Check sheet for the modelled part. Datum: model origin and axes. Units: mm. A direction names the side the tool comes from. Give positions to 0.01 mm unless a question says otherwise; leave off trailing zeros. Order: outer loops, then holes, each group sorted by start corner. A loop starts at its lowest first (then second) coordinate and runs counter-clockwise, first axis right, second up.
```python
from build123d import *

# Parameters (mm, degrees)
F0_W          = 16.5
F0_H          = 11
F1_DEPTH      = 10
F2_W          = 5
F2_H          = 11
F3_DEPTH      = 21
F4_R          = 1.1
F5_DEPTH      = 25
F6_W          = 1.5
F6_H          = 11
F7_DEPTH      = 21
F8_DEPTH      = 25.75
F9_W          = 13
F9_H          = 10
F10_DEPTH     = 10
F11_R         = 3
F12_DEPTH     = 3.5
F13_R         = 1.45
F14_DEPTH     = 25
F15_R         = 1
F16_T1_DEPTH  = 11
F16_S5_W      = 1
F16_S5_H      = 1
F16_T6_DEPTH  = 1
F16_S11_W     = 1
F16_S11_H     = 1
F16_T12_DEPTH = 1


# Not quite as in the source:
# - a fillet or chamfer that OpenCascade refuses, or shapes differently, is made with other operations: its cross-section is extruded or revolved along the edge and cut away or added


with BuildPart() as f1:
    # F0 (on Front) → F1 (new body)
    with BuildSketch(Plane.XZ):
        with Locations((8.25, 5.5)):
            Rectangle(F0_W, F0_H)
    extrude(amount=F1_DEPTH)

    # F2 (on face) → F3 (join)
    with BuildSketch(Plane.XZ.offset(10)):
        with Locations((14, 5.5)):
            Rectangle(F2_W, F2_H)
        with Locations((2.5, 5.5)):
            Rectangle(F2_W, F2_H)
    extrude(amount=F3_DEPTH)

    # F4 (on face) → F5 (cut)
    with BuildSketch(Plane(origin=(0, 0, 0), x_dir=(0, -1, 0), z_dir=(-1, 0, 0))):
        with BuildLine():
            ThreePointArc((24.9, 8), (26, 6.9), (27.1, 8))
            Line((27.1, 8), (26, 8))
            Line((26, 8), (24.9, 8))
        make_face()
        with BuildLine():
            Line((26, 8), (27.1, 8))
            ThreePointArc((27.1, 8), (26, 9.1), (24.9, 8))
            Line((24.9, 8), (26, 8))
        make_face()
        with Locations((16.5, 8)):
            Circle(F4_R)
    extrude(amount=-F5_DEPTH, mode=Mode.SUBTRACT)

    # F6 (on face) → F7 (cut)
    with BuildSketch(Plane.XZ.offset(31)):
        with Locations((0.75, 5.5)):
            Rectangle(F6_W, F6_H)
    extrude(amount=-F7_DEPTH, mode=Mode.SUBTRACT)

    # F8 (add): a face of the model
    f8_faces = [f1.faces().sort_by_distance(p)[0] for p in [
        (0, -5, 5.5),
    ]]
    extrude(f8_faces, amount=F8_DEPTH)

    # F9 (on face) → F10 (join)
    with BuildSketch(Plane.XY.offset(11)):
        with Locations((-19.25, -5)):
            Rectangle(F9_W, F9_H)
    extrude(amount=F10_DEPTH)

    # F11 (on face) → F12 (cut)
    with BuildSketch(Plane(origin=(0, 0, 0), x_dir=(-1, 0, 0), z_dir=(0, 1, 0))):
        with BuildLine():
            ThreePointArc((22.25, 15.75), (21.3713203436, 17.8713203436), (19.25, 18.75))
            Line((19.25, 18.75), (19.25, 12.75))
            ThreePointArc((19.25, 12.75), (21.3713203436, 13.6286796564), (22.25, 15.75))
        make_face()
        with BuildLine():
            Line((19.25, 12.75), (19.25, 18.75))
            ThreePointArc((19.25, 18.75), (16.25, 15.75), (19.25, 12.75))
        make_face()
        with Locations((19.25, 5.25)):
            Circle(F11_R)
    extrude(amount=-F12_DEPTH, mode=Mode.SUBTRACT)

    # F13 (on face) → F14 (cut)
    with BuildSketch(Plane(origin=(0, 0, 0), x_dir=(-1, 0, 0), z_dir=(0, 1, 0))):
        with Locations((19.25, 15.75)):
            Circle(F13_R)
        with Locations((19.25, 5.25)):
            Circle(F13_R)
    extrude(amount=-F14_DEPTH, mode=Mode.SUBTRACT)

    # F15
    f15_edges = [f1.edges().sort_by_distance(p)[0] for p in [
        (-12.75, -5, 21),
        (-25.75, -5, 21),
        (-19.25, 0, 21),
        (-25.75, 0, 10.5),
        (-25.75, -10, 10.5),
        (-25.75, -5, 0),
        (-4.625, 0, 0),
        (-12.125, -10, 0),
        (-12.75, 0, 16),
        (-12.75, -10, 16),
        (1.875, 0, 11),
        (-5.625, -10, 11),
        (8.25, -10, 11),
        (8.25, -10, 0),
        (3.25, -31, 11),
        (14, -31, 11),
        (14, -31, 0),
        (16.5, -15.5, 0),
        (3.25, -31, 0),
    ]]
    fillet(f15_edges, radius=F15_R)

    # F16: fillet of radius 1 on 1 edges, made by hand

    # F16_s2 → F16_t1 (cut)
    with BuildSketch(Plane.YZ.offset(-24.75)):
        with BuildLine():
            ThreePointArc((-10, 20), (-9.7071067812, 20.7071067812), (-9, 21))
            Line((-9, 21), (-10, 21))
            Line((-10, 21), (-10, 20))
        make_face()
    extrude(amount=F16_T1_DEPTH, mode=Mode.SUBTRACT)


with BuildPart() as f16_tool4:
    # F16_s5 → F16_t6 (new body)
    with BuildSketch(Plane.XZ.offset(9)):
        with Locations((-25.25, 20.5)):
            Rectangle(F16_S5_W, F16_S5_H)
    extrude(amount=F16_T6_DEPTH)

    # F16_s7 → F16_t8 (revolve, cut)
    with BuildSketch(Plane(origin=(-24.75, -9, 20), x_dir=(0.7071067812, 0, -0.7071067812), z_dir=(-0.7071067812, 0, -0.7071067812))):
        with BuildLine():
            ThreePointArc((0, -1), (1, 0), (0, 1))
            Line((0, 1), (0, -1))
        make_face()
    revolve(axis=Axis((-24.75, -9, 20), (0, -1, 0)), mode=Mode.SUBTRACT)


with BuildPart() as f1_1:
    add(f1.part)

    # F16_t3: cut F16_tool4
    add(f16_tool4.part, mode=Mode.SUBTRACT)


with BuildPart() as f16_tool10:
    # F16_s11 → F16_t12 (new body)
    with BuildSketch(Plane.XZ.offset(9)):
        with Locations((-13.25, 20.5)):
            Rectangle(F16_S11_W, F16_S11_H)
    extrude(amount=F16_T12_DEPTH)

    # F16_s13 → F16_t14 (revolve, cut)
    with BuildSketch(Plane(origin=(-13.75, -9, 20), x_dir=(-0.7071067812, 0, -0.7071067812), z_dir=(-0.7071067812, 0, 0.7071067812))):
        with BuildLine():
            ThreePointArc((0, -1), (1, 0), (0, 1))
            Line((0, 1), (0, -1))
        make_face()
    revolve(axis=Axis((-13.75, -9, 20), (0, -1, 0)), mode=Mode.SUBTRACT)


with BuildPart() as f1_2:
    add(f1_1.part)

    # F16_t9: cut F16_tool10
    add(f16_tool10.part, mode=Mode.SUBTRACT)


solid = f1_2.part
```
(1) Cross-section at D-D on y = -2. Enter the section's corners in (x, z), then the cut area to 3 significant figures.
Response values:
outline: (-25.75, 1) arc R1 ccw to (-24.75, 0) - (15.5, 0) arc R1 ccw to (16.5, 1) - (16.5, 11) - (-12.75, 11) - (-12.75, 20) arc R1 ccw to (-13.75, 21) - (-24.75, 21) arc R1 ccw to (-25.75, 20) - close; hole circle Ø6 at (-19.25, 5.25); hole circle Ø6 at (-19.25, 15.75)
area: 537 mm2
(2) Release check for a two-part mould opening along Y. For faces 4 (the face through (3.274, -30.699, 10.715)), 5 (the face through (3.23, -15.63, 7.33)), 6 (the face through (-21, -3.5, 6)) record: released by +Y, released by -Y, zero draft, split by the parting line, or undercut.
Response values:
face 4: released by -Y
face 5: undercut
face 6: released by +Y
(3) Cross-section at A-A on z = 5.25. Enter the section's corners in (x, y).
Response values:
outline: (-25.75, -9) arc R1 ccw to (-24.75, -10) - (-20.7, -10) - (-20.7, -3.5) - (-22.25, -3.5) - (-22.25, 0) - (-24.75, 0) arc R1 ccw to (-25.75, -1) - close; (-17.8, -10) - (1.5, -10) - (1.5, -31) - (5, -31) - (5, -10) - (11.5, -10) - (11.5, -31) - (16.5, -31) - (16.5, 0) - (-16.25, 0) - (-16.25, -3.5) - (-17.8, -3.5) - close
(4) Gauge pin test, flat ends, axial feed: pin 1 Ø1.5 at (x, z) = (-2.5, 12) entering from +Y; pin 2 Ø12 at (y, z) = (-15.5, 2.5) entering from -X; pin 3 Ø12 at (x, y) = (7, -17) entering from +Z; pin 4 Ø3 at (x, z) = (8.5, 7) entering from -Y. Record the tip position at first contact, or that the pin passes through.
Response values:
pin 1: passes through
pin 2: stops at x = -25.62
pin 3: stops at z = 11
pin 4: stops at y = -10
(5) Cross-section at C-C on x = 3.5. Enter the section's corners in (y, z), then the cut area to 3 significant figures.
Response values:
outline: (-31, 1) arc R1 ccw to (-30, 0) - (-1, 0) arc R1 ccw to (0, 1) - (0, 10) arc R1 ccw to (-1, 11) - (-30, 11) arc R1 ccw to (-31, 10) - close; hole circle Ø2.2 at (-26, 8); hole circle Ø2.2 at (-16.5, 8)
area: 333 mm2
(6) Set-up check for faces 1 (the face through (5.33, -8.85, 11)), 2 (the face through (8.296, -9.699, 0.285)), 3 (the face through (-13.051, -0.285, 15.07)): record each of +Z, -Z, +X, -X, +Y, -Y from which the full face is reachable in a straight line by a thin tool's end or side.
Response values:
face 1: +Z, +X, +Y, -Y
face 2: -Z, -Y
face 3: +Z, +X, +Y
(7) Cross-section at B-B on y = -26. Enter the section's corners in (x, z).
Response values:
outline: (1.5, 0) - (5, 0) - (5, 6.9) - (1.5, 6.9) - close; (1.5, 9.1) - (5, 9.1) - (5, 11) - (1.5, 11) - close; (11.5, 0) - (15.5, 0) arc R1 ccw to (16.5, 1) - (16.5, 6.9) - (11.5, 6.9) - close; (11.5, 9.1) - (16.5, 9.1) - (16.5, 11) - (11.5, 11) - close
(8) Material ranges on L1, parallel to X at y = -17.5, z = 2.25; L2, parallel to Z at x = -19.25, y = -5.25; L3, parallel to Z at x = 14, y = -26, recorded low to high.
Response values:
L1: x = 1.5 to 5, 11.5 to 16.5
L2: z = 0 to 3.8, 6.7 to 14.3, 17.2 to 21
L3: z = 0 to 6.9, 9.1 to 11
